Check sheet for the drawn part. Datum: minimum x, y, z corner. Units: mm. A direction names the side the tool comes from. Round coordinates to 2 decimals unless told otherwise and drop trailing zeros. Write each loop counter-clockwise with the first axis right and the second up, starting at its lowest first coordinate (ties: lowest second). Pieces come first, ordered by that corner, then holes. Notation, with made-up numbers: M 47,38 L 78,38 A24 ccw 78,50 Z; hole C 62,-31 d4. An arc over 180 degrees is marked long. Use a Markdown table: item, result.
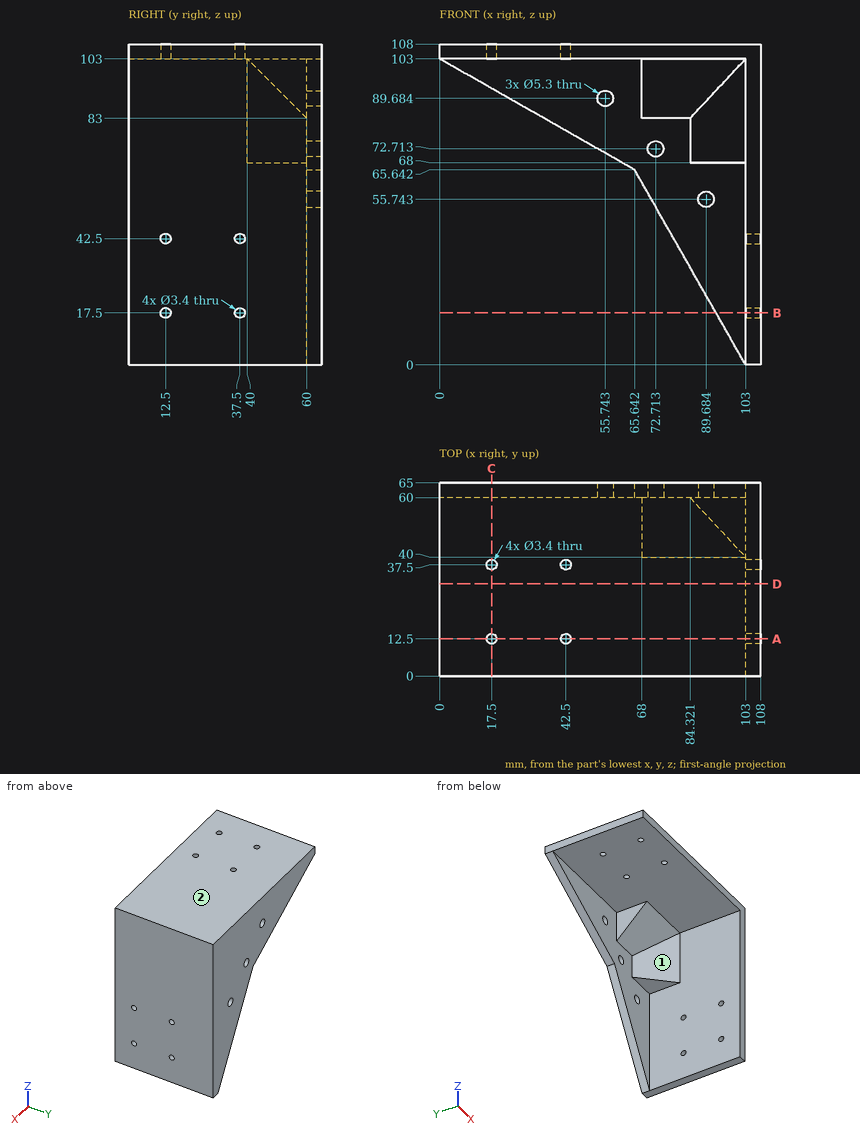
Item 1: Cross-section at B-B, the plane z = 17.5. Record the cut outline in (x, y).
Outcome:
| item | result |
|---|---|
| outline | M 93.04,60 L 103,60 L 103,39.2 L 108,39.2 L 108,65 L 93.04,65 Z; M 103,0 L 108,0 L 108,10.8 L 103,10.8 Z; M 103,14.2 L 108,14.2 L 108,35.8 L 103,35.8 Z |
Item 2: Cross-section at D-D, the plane y = 31. Record the cut outline in (x, z).
Outcome:
| item | result |
|---|---|
| outline | M 0,103 L 103,103 L 103,0 L 108,0 L 108,108 L 0,108 Z |
Item 3: Material ranges on line 1 along Y through (x, z) = (17.5, 105.3); line 2 along X through (y, z) = (37, 104) (1 decimal); line 3 along Z through (x, y) = (60, 57.5), recorded low to high. Write a range as from..to.
Outcome:
| item | result |
|---|---|
| line 1 | y = 0..10.8, 14.2..35.8, 39.2..65 |
| line 2 | x = 0..15.9, 19.1..40.9, 44.1..108 |
| line 3 | z = 103..108 |
Item 4: Cross-section at A-A, the plane y = 12.5. Record the cut outline in (x, z), and give its area (3 significant figures).
Outcome:
| item | result |
|---|---|
| outline | M 0,103 L 15.8,103 L 15.8,108 L 0,108 Z; M 19.2,103 L 40.8,103 L 40.8,108 L 19.2,108 Z; M 44.2,103 L 103,103 L 103,44.2 L 108,44.2 L 108,108 L 44.2,108 Z; M 103,0 L 108,0 L 108,15.8 L 103,15.8 Z; M 103,19.2 L 108,19.2 L 108,40.8 L 103,40.8 Z |
| area | 987 mm2 |
Item 5: Access from +Z, -Z, +X, -X, +Y, -Y to the whole of each face (thin tool, end or side, straight path). Record for the marked faces 1 and 2.
Outcome:
| item | result |
|---|---|
| face 1 | -Z, -X, -Y |
| face 2 | +Z, +X, -X, +Y, -Y |
Item 6: Cross-section at C-C, the plane x = 17.5. Record the cut outline in (y, z).
Outcome:
| item | result |
|---|---|
| outline | M 0,103 L 10.8,103 L 10.8,108 L 0,108 Z; M 14.2,103 L 35.8,103 L 35.8,108 L 14.2,108 Z; M 39.2,103 L 60,103 L 60,93.04 L 65,93.04 L 65,108 L 39.2,108 Z |
Item 7: Go/stop test with flat-tipped pins: pin 1 (8 mm diameter, centred on y = 46, z = 13.5, fed in from -X); pin 2 (22 mm diameter, centred on y = 45, z = 89, fed in from -X); pin 3 (7 mm diameter, centred on x = 55.74, z = 89.68, fed in from -Y). Record where each tip stops, or that it passes through.
Outcome:
| item | result |
|---|---|
| pin 1 | stops at x = 103 |
| pin 2 | stops at x = 68 |
| pin 3 | stops at y = 60 |
